```python
from build123d import *

# Parameters (mm, degrees)
F1_W     = 44.45
F1_H     = 19.05
F2_DEPTH = 63.5
F3_DEPTH = 19.05
F5_DEPTH = 19.05


with BuildPart() as f2:
    # F1 (on face) → F2 (new body)
    with BuildSketch(Plane.YZ):
        with Locations((22.225, 18.076053)):
            Rectangle(F1_W, F1_H)
    extrude(amount=-F2_DEPTH)

    # F0 (on Right) → F3 (join)
    with BuildSketch(Plane.YZ):
        Polygon((42.11467, 52.503103), (23.06467, 52.503103), (-21.38533, 20.753103), (-21.38533, 8.053103), (42.11467, 8.053103), align=None)
    extrude(amount=F3_DEPTH)

    # F4 (on face) → F5 (join)
    with BuildSketch(Plane(origin=(-63.5, 0, 0), x_dir=(0, -1, 0), z_dir=(-1, 0, 0))):
        Polygon((-23.505, 52.787023), (-42.553797, 53.001053), (-42.553797, 8.551053), (20.946203, 8.551053), (20.946203, 21.251053), align=None)
    extrude(amount=F5_DEPTH)


solid = f2.part
```
For this review, take the finished solid that the model builds, in its own axes (mm). A direction names the side the tool comes from. Round coordinates to 2 decimals unless told otherwise and drop trailing zeros. Write each loop counter-clockwise with the first axis right and the second up, starting at its lowest first coordinate (ties: lowest second). Pieces come first, ordered by that corner, then holes. Notation, with made-up numbers: (3, 72.5) - (11, 72.5) arc R37 ccw to (11, 108.5) - close; hole circle Ø7 at (37, 61). An arc over 180 degrees is marked (long way). Put each result on its own line as item: value.
Q1. Mouldability with a two-part tool opening along X and no side actions: class faces 1 (the face through (-82.55, 18, 26)), 2 (the face through (-31, 0, 18)), 3 (the face through (0, 43, 18)), 4 (the face through (-73, 42.554, 31)) as released by +X, released by -X, zero draft, split by the parting line, or undercut.
Solved:
face 1: released by -X
face 2: undercut
face 3: released by +X
face 4: zero draft
Q2. We need section A-A (z = 46.5). Give the boundary of the cut face in (x, y), and give its area (3 significant figures).
Solved:
outline: (-82.55, 14.64) - (-63.5, 14.64) - (-63.5, 42.55) - (-82.55, 42.55) - close; (0, 14.66) - (19.05, 14.66) - (19.05, 42.11) - (0, 42.11) - close
area: 1,050 mm2
Q3. Machinability: for faces 5 (the face through (-63.5, 11, 31)), 6 (the face through (-73, -20.946, 15)), 7 (the face through (-31, 22, 27.601)), 8 (the face through (9.39, 1.15, 36.85)), 9 (the face through (9, 42.115, 30)), which of the approach directions +Z, -Z, +X, -X, +Y, -Y give a long, thin tool a straight path to every point of the face, cutting with its end or side? Answer none if there is none.
Solved:
face 5: +Z, -Y
face 6: +Z, -Z, -X, -Y
face 7: +Z, +Y, -Y
face 8: +Z, +X, -Y
face 9: +Z, -Z, +X, +Y
Q4. Insertion check: pin 1 Ø9.5 at (x, y) = (13, 29) entering from +Z; pin 2 Ø15 at (x, z) = (5, 35.5) entering from +Y; pin 3 Ø1.5 at (y, z) = (43.5, 19.5) entering from -X. Each pin has a flat end and moves straight along its axis. Give the tip position at first contact, or say it passes through.
Solved:
pin 1: stops at z = 52.5
pin 2: stops at y = 42.11
pin 3: stops at x = -63.5
Q5. We need section B-B (x = 5.5). Give the boundary of the cut face in (y, z), and give its area (3 significant figures).
Solved:
outline: (-21.39, 8.05) - (42.11, 8.05) - (42.11, 52.5) - (23.06, 52.5) - (-21.39, 20.75) - close
area: 2,120 mm2
Q6. We need section C-C (y = 16.5). Give the boundary of the cut face in (x, z).
Solved:
outline: (-82.55, 8.55) - (0, 8.55) - (0, 8.05) - (19.05, 8.05) - (19.05, 47.81) - (0, 47.81) - (0, 27.6) - (-63.5, 27.6) - (-63.5, 47.82) - (-82.55, 47.82) - close
Q7. We need section D-D (z = 16). Give the boundary of the cut face in (x, y).
Solved:
outline: (-82.55, -20.95) - (-63.5, -20.95) - (-63.5, 0) - (0, 0) - (0, -21.39) - (19.05, -21.39) - (19.05, 42.11) - (0, 42.11) - (0, 44.45) - (-63.5, 44.45) - (-63.5, 42.55) - (-82.55, 42.55) - close
Q8. Wall thickness on probe 1 along X at (y, z) = (-17.5, 16.5); probe 2 along Z at (x, y) = (-4.5, 23); probe 3 along Y at (x, z) = (-28.5, 27): over which ranges is each line inside the solid? List them lowest first.
Solved:
probe 1: x = -82.55 to -63.5, 0 to 19.05
probe 2: z = 8.55 to 27.6
probe 3: y = 0 to 44.45
